The drawing under review shows one solid part. Ordinate dimensions are in mm from its lowest x, y, z. A direction names the side the tool comes from. Round coordinates to 2 decimals unless told otherwise and drop trailing zeros. Order: outer loops, then holes, each group sorted by start corner. A loop starts at its lowest first (then second) coordinate and runs counter-clockwise, first axis right, second up. Notation, with made-up numbers: M 71.25,-20.75 L 99.25,-20.75 A20 ccw 99.25,18.25 Z; hole C 31.25,80.25 d10. An arc over 180 degrees is marked long. Answer as a JSON object with one key per item and string values.
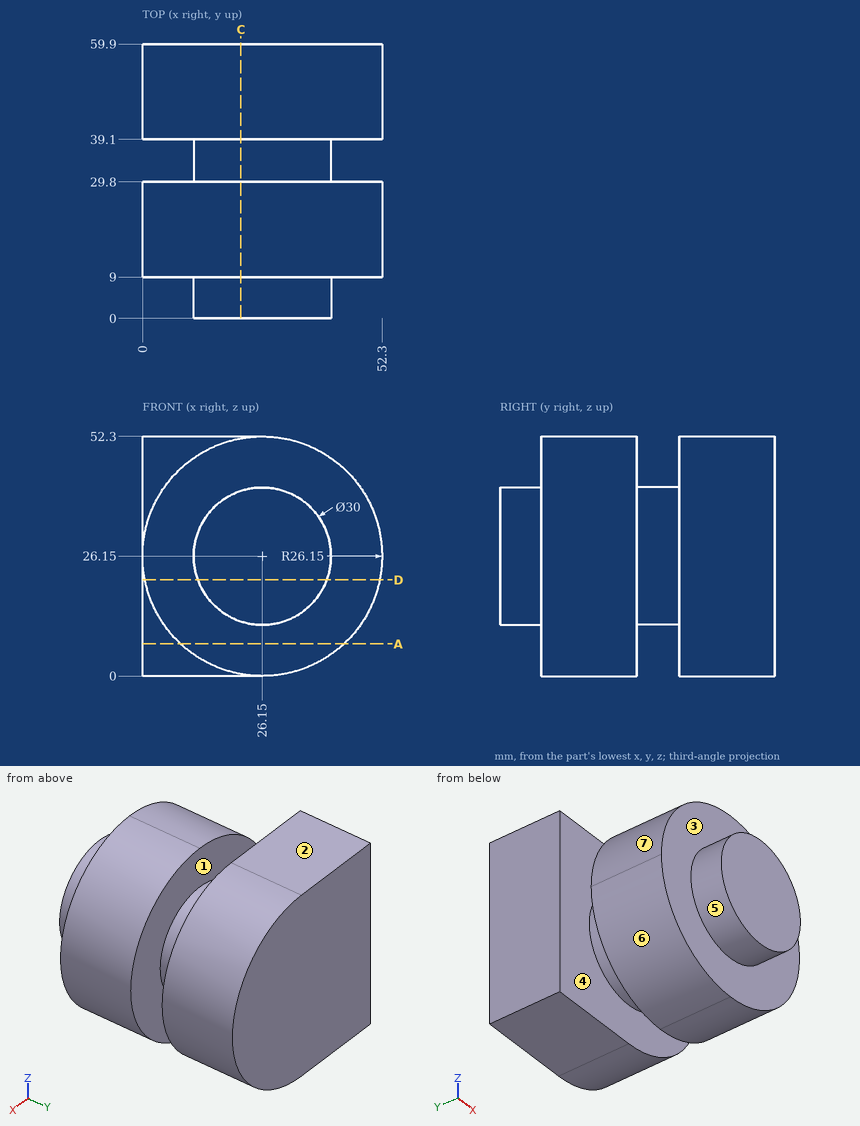
1) Add section C-C on x = 21.5. State the section outline as (y, z) points, and give its area (3 significant figures).
Geometry check:
{"outline": "M 0,11.89 L 9,11.89 L 9,0.42 L 29.8,0.42 L 29.8,11.89 L 39.1,11.89 L 39.1,0 L 59.9,0 L 59.9,52.3 L 39.1,52.3 L 39.1,40.41 L 29.8,40.41 L 29.8,51.88 L 9,51.88 L 9,40.41 L 0,40.41 Z", "area": "2,680 mm²"}
2) Add section D-D on z = 21. State the section outline as (x, y) points, and give its area (3 significant figures).
Geometry check:
{"outline": "M 0,39.1 L 12.06,39.1 L 12.06,29.8 L 0.51,29.8 L 0.51,9 L 12.06,9 L 12.06,0 L 40.24,0 L 40.24,9 L 51.79,9 L 51.79,29.8 L 40.24,29.8 L 40.24,39.1 L 51.79,39.1 L 51.79,59.9 L 0,59.9 Z", "area": "2,660 mm²"}
3) For L1, parallel to Y at x = 45.5, z = 34.5; L2, parallel to X at y = 38, z = 30; L3, parallel to Z at x = 36, y = 35, list the stretches that pass through material, from the lowest coordinate up.
Geometry check:
{"L1": "y = 9 to 29.8, 39.1 to 59.9", "L2": "x = 11.65 to 40.65", "L3": "z = 14.84 to 37.46"}
4) Insertion check: P1, Ø6, axis at y = 25, z = 10, coming from the +X side; P2, Ø2, axis at x = 33, z = 11, coming from the -Y side; P3, Ø3, axis at y = 8, z = 6, coming from the -X side. Each pin has a flat end and moves straight along its axis. Give the tip position at first contact, or say it passes through.
Geometry check:
{"P1": "stops at x = 48.75", "P2": "stops at y = 9", "P3": "stops at x = 8.22"}
5) Add section A-A on z = 7. State the section outline as (x, y) points.
Geometry check:
{"outline": "M 0,39.1 L 43.96,39.1 L 43.96,59.9 L 0,59.9 Z; M 8.34,9 L 43.96,9 L 43.96,29.8 L 8.34,29.8 Z"}
6) Mouldability with a two-part tool opening along Y and no side actions: class the marked faces 1, 2, 3 and 4 as +Y half, -Y half, draft (parallel to the pull), parting line (faces both ways), or undercut.
Geometry check:
{"face 1": "undercut", "face 2": "draft", "face 3": "-Y half", "face 4": "undercut"}
7) Machinability: for the marked faces 5, 6 and 7, which of the approach directions +Z, -Z, +X, -X, +Y, -Y give a long, thin tool a straight path to every point of the face, cutting with its end or side? Answer none if there is none.
Geometry check:
{"face 5": "-Y", "face 6": "-Z, -X, -Y", "face 7": "+Z, -X, -Y"}
